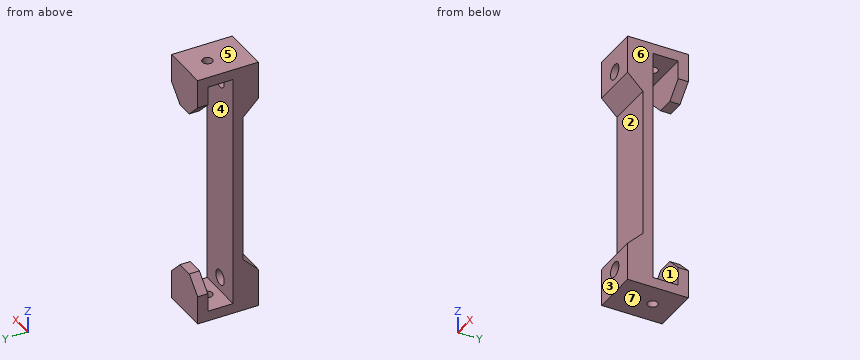
```python
from build123d import *

# Parameters (mm, degrees)
F1_DEPTH = 7
F2_SIZE  = 4.49999
F3_R     = 2.25
F4_DEPTH = 7.5
F5_R     = 1.5
F6_DEPTH = 76.001


# Not quite as in the source:
# - a fillet or chamfer is up to 0.001 mm smaller than in the source, because OpenCascade refuses the exact size


with BuildPart() as f1:
    # F0 (on Right) → F1 (new body, symmetric)
    with BuildSketch(Plane.YZ):
        Polygon((-3.75, 35), (3.75, 35), (3.75, 25), (6.75, 25), (6.75, 38), (-11.25, 38), (-11.25, 26.71), (-6.75, 26.71), (-6.75, -26.71), (-11.25, -26.71), (-11.25, -38), (6.75, -38), (6.75, -25), (3.75, -25), (3.75, -35), (-3.75, -35), align=None)
    extrude(amount=F1_DEPTH, both=True)

    # F2 (size 4.5 in the source; OpenCascade refuses exactly that, so slightly less here)
    f2_edges = [f1.edges().sort_by_distance(p)[0] for p in [
        (0, -6.75, 26.71),
        (0, -6.75, -26.71),
        (-7, 5.25, 25),
        (7, 5.25, 25),
        (-7, 5.25, -25),
        (7, 5.25, -25),
    ]]
    chamfer(f2_edges, length=F2_SIZE)

    # F3 (on face) → F4 (cut, through all)
    with BuildSketch(Plane.XZ.offset(11.25)):
        with Locations((0, 30.855)):
            Circle(F3_R)
        with Locations((0, -30.855)):
            Circle(F3_R)
    extrude(amount=-F4_DEPTH, mode=Mode.SUBTRACT)

    # F5 (on face) → F6 (cut, through all)
    with BuildSketch(Plane.XY.offset(38)):
        Circle(F5_R)
    extrude(amount=-F6_DEPTH, mode=Mode.SUBTRACT)


solid = f1.part
```
The listing builds one solid part. Answer for the finished solid, in the listing's coordinates (mm). Face numbers are marked on the shaded views. A direction names the side the tool comes from. Give positions to 0.01 mm unless a question says otherwise; leave off trailing zeros. Order: outer loops, then holes, each group sorted by start corner. A loop starts at its lowest first (then second) coordinate and runs counter-clockwise, first axis right, second up. Notation, with made-up numbers: (57.5, -5) - (76.5, -5) arc R30 ccw to (76.5, 23) - close; hole circle Ø11 at (15, 46). An arc over 180 degrees is marked (long way). Answer in a Markdown table with one row per item. Add a question column.
Q1. The part is cut by section D-D (y = 0). Determine the outline of the cut face in (x, z).
Q2. The part is cut by section C-C (y = -8.5). Determine the outline of the cut face in (x, z) (3 decimals).
Q3. Which of the six approach directions +Z, -Z, +X, -X, +Y, -Y give full straight-line access (tool end or side, diameter ignored) to the marked faces 1, 2 and 3?
Q4. The part is cut by section B-B (x = 0). Give the number of separate pieces and of enclosed holes in the cut face, then the cut area to 3 significant figures.
Q5. Given P1, Ø1.5, axis at x = 1.5, z = -21.5, coming from the -Y side; P2, Ø3, axis at x = -3, z = -19, coming from the -Y side; P3, Ø8, axis at x = 1, z = -20, coming from the -Y side, each flat-ended and moving along its own axis, determine where each tip first touches the part or whether it passes through.
Q6. The part is cut by section A-A (y = 4.5). Determine the outline of the cut face in (x, z).
Q7. Find the intervals of material crossed by line 1 along Z through (x, y) = (0, -5.25) (3 decimals); line 2 along Z through (x, y) = (-0.25, 5.5); line 3 along Z through (x, y) = (-2.75, 3.5), in increasing order. Write a range as [from, to].
Q8. For a pull along Z with two mould halves and no side action, classify the marked faces 4, 5, 6 and 7 as released by +Z, released by -Z, zero draft, split by the parting line, or undercut.
Determined:
| question | item | result |
|---|---|---|
| 1 | outline | (-7, -38) - (-1.5, -38) - (-1.5, -35) - (-7, -35) - close; (-7, 35) - (-1.5, 35) - (-1.5, 38) - (-7, 38) - close; (1.5, -38) - (7, -38) - (7, -35) - (1.5, -35) - close; (1.5, 35) - (7, 35) - (7, 38) - (1.5, 38) - close |
| 2 | outline | (-7, -38) - (7, -38) - (7, -23.96) - (-7, -23.96) - close; (-7, 23.96) - (7, 23.96) - (7, 38) - (-7, 38) - close; hole circle Ø4.5 at (0, -30.855); hole circle Ø4.5 at (0, 30.855) |
| 3 | face 1 | +X, -X |
| 3 | face 2 | +X, -X, -Y |
| 3 | face 3 | +Z, -Z, +X, -X, -Y |
| 4 | separate pieces | 5 |
| 4 | enclosed holes | 0 |
| 4 | area | 387 mm² |
| 5 | P1 | stops at y = -6.79 |
| 5 | P2 | stops at y = -6.75 |
| 5 | P3 | stops at y = -8.54 |
| 6 | outline | (-7, -38) - (7, -38) - (7, -29.5) - (2.5, -25) - (-2.5, -25) - (-7, -29.5) - close; (-7, 29.5) - (-2.5, 25) - (2.5, 25) - (7, 29.5) - (7, 38) - (-7, 38) - close |
| 7 | line 1 | z = [-38, -33.105], [-28.605, 28.605], [33.105, 38] |
| 7 | line 2 | z = [-38, -25], [25, 38] |
| 7 | line 3 | z = [-38, -35], [35, 38] |
| 8 | face 4 | undercut |
| 8 | face 5 | released by +Z |
| 8 | face 6 | zero draft |
| 8 | face 7 | released by -Z |
